The figure shows three views and two pictorial views of one solid part (mm, origin at its lowest corner). Answer the questions. Round coordinates to 2 decimals unless told otherwise and drop trailing zeros. Loops run counter-clockwise (first coordinate to the right, second up) from the corner with the lowest first, then second, coordinate; pieces in that order, holes last. Notation, with made-up numbers: (37.25, 57.25) -> (54.25, 57.25) arc R24 cw to (54.25, 93.25) -> close; hole circle Ø4 at (-22.5, 32.5). An arc over 180 degrees is marked (long way). Put each result on its own line as item: value.
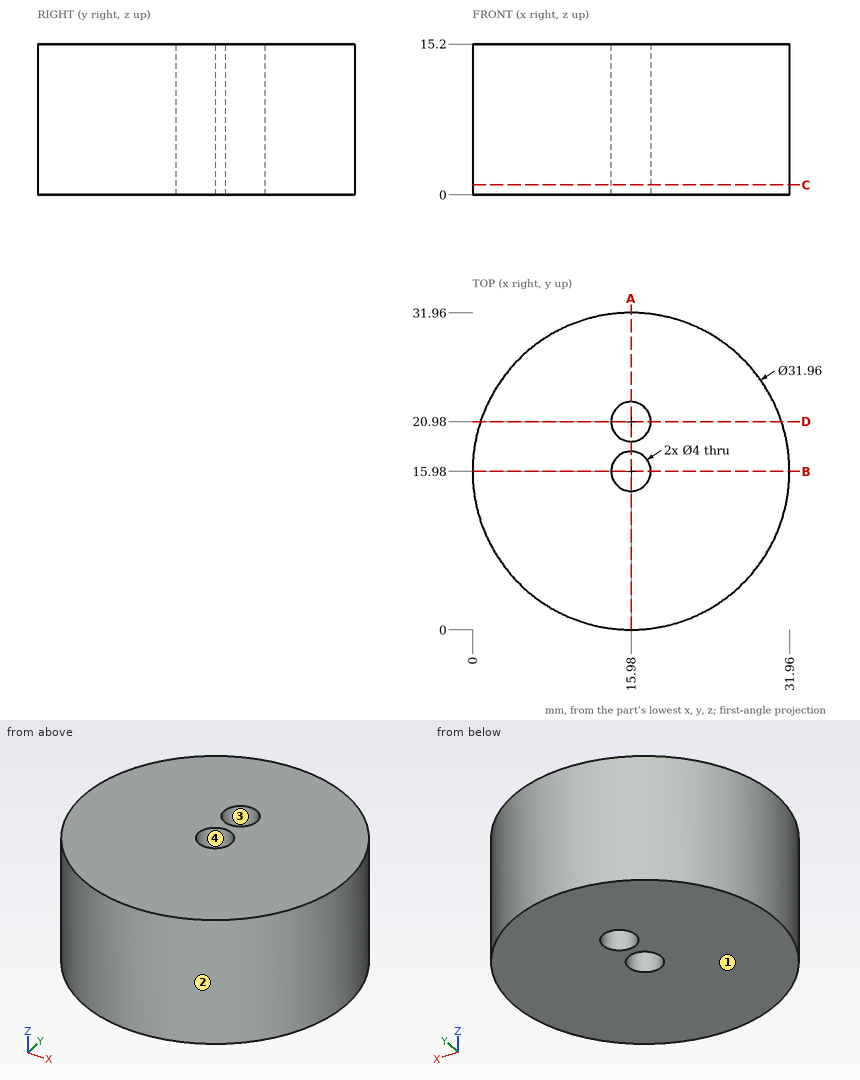
Item 1: The part is cut by section B-B (y = 15.98). Determine the outline of the cut face in (x, z).
Derived:
outline: (0, 0) -> (13.98, 0) -> (13.98, 15.2) -> (0, 15.2) -> close; (17.98, 0) -> (31.96, 0) -> (31.96, 15.2) -> (17.98, 15.2) -> close
Item 2: The part is cut by section C-C (z = 1). Determine the outline of the cut face in (x, y), then the cut area to 3 significant figures.
Derived:
outline: circle Ø31.96 at (15.98, 15.98); hole circle Ø4 at (15.98, 15.98); hole circle Ø4 at (15.98, 20.98)
area: 777 mm^2
Item 3: The part is cut by section A-A (x = 15.98). Determine the outline of the cut face in (y, z), then the cut area to 3 significant figures.
Derived:
outline: (0, 0) -> (13.98, 0) -> (13.98, 15.2) -> (0, 15.2) -> close; (17.98, 0) -> (18.98, 0) -> (18.98, 15.2) -> (17.98, 15.2) -> close; (22.98, 0) -> (31.96, 0) -> (31.96, 15.2) -> (22.98, 15.2) -> close
area: 364 mm^2
Item 4: Flat-ended cylindrical pins translate along their axes: pin 1 Ø4 at (y, z) = (3.5, 8) entering from -X; pin 2 Ø2.5 at (x, y) = (15.98, 20.98) entering from +Z; pin 3 Ø5 at (x, z) = (24.5, 2) entering from +Y; pin 4 Ø2 at (y, z) = (21, 13.5) entering from -X. Find the tip coordinate at first contact, or state that the pin passes through.
Derived:
pin 1: stops at x = 3.92
pin 2: passes through
pin 3: stops at y = 30.78
pin 4: stops at x = 0.51
Item 5: Find the intervals of material crossed by line 1 along Y through (x, z) = (15.98, 3.5); line 2 along X through (y, z) = (16.5, 2.75); line 3 along Y through (x, z) = (15.5, 4.25), in increasing order.
Derived:
line 1: y = 0 to 13.98, 17.98 to 18.98, 22.98 to 31.96
line 2: x = 0.01 to 14.05, 17.91 to 31.95
line 3: y = 0.01 to 14.04, 17.92 to 19.04, 22.92 to 31.95
Item 6: The part is cut by section D-D (y = 20.98). Determine the outline of the cut face in (x, z).
Derived:
outline: (0.8, 0) -> (13.98, 0) -> (13.98, 15.2) -> (0.8, 15.2) -> close; (17.98, 0) -> (31.16, 0) -> (31.16, 15.2) -> (17.98, 15.2) -> close
Item 7: For a pull along Y with two mould halves and no side action, classify the marked faces 1, 2, 3 and 4 as pulls with the +Y half, pulls with the -Y half, needs draft (parallel to the pull), parting line crosses it, or undercut.
Derived:
face 1: needs draft
face 2: parting line crosses it
face 3: undercut
face 4: undercut
